Verification items for the finished model (mm, model axes). A direction names the side the tool comes from. Coordinates: 2 decimals unless noted, no trailing zeros. Write each loop counter-clockwise with the first axis right and the second up, starting at its lowest first coordinate (ties: lowest second). Pieces come first, ordered by that corner, then holes. Notation, with made-up numbers: (79, 7) -> (94, 7) arc R7 ccw to (94, 14) -> close; hole circle Ø4 at (8, -2). An arc over 180 degrees is marked (long way). Answer in a Markdown table with one row per item.
```python
from build123d import *

# Parameters (mm, degrees)
SKETCH1_R           = 1.3462
SKETCH1_W           = 3.7846
SKETCH1_H           = 52.6961
BOSS_EXTRUDE1_DEPTH = 3.048
SKETCH2_R           = 1.524
CUT_EXTRUDE1_DEPTH  = 430.898988368


with BuildPart() as part:
    # Sketch1 → Boss-Extrude1 (new body)
    # profile 1 of 3: a face of its own
    with BuildSketch(Plane.XY):
        with BuildLine():
            Line((-401.0571, 150.956597849), (-401.0571, 148.341))
            Line((-401.0571, 148.341), (-399.1521, 148.341))
            Line((-399.1521, 148.341), (-395.3675, 148.341))
            Line((-395.3675, 148.341), (-395.3675, 149.2432))
            Line((-395.3675, 149.2432), (-309.8086, 149.2432))
            Line((-309.8086, 149.2432), (-309.8086, 128.8851))
            Line((-309.8086, 128.8851), (-305.87795, 128.8851))
            Line((-305.87795, 128.8851), (-301.9473, 132.81575))
            Line((-301.9473, 132.81575), (-301.9473, 150.9704))
            ThreePointArc((-301.9473, 150.9704), (-303.063223164, 153.664476836), (-305.7573, 154.7804))
            Line((-305.7573, 154.7804), (-397.247125, 154.7804))
            ThreePointArc((-397.247125, 154.7804), (-399.946077222, 153.659592612), (-401.0571, 150.956597849))
        make_face()
        with Locations(Location((-397.247125, 150.9704, 0), (0, 0, 180))):
            Circle(SKETCH1_R, mode=Mode.SUBTRACT)
        with Locations(Location((-305.7573, 150.9704, 0), (0, 0, 180))):
            Circle(SKETCH1_R, mode=Mode.SUBTRACT)
    # profile 2 of 3: a face of its own
    with BuildSketch(Plane.XY):
        with Locations((-397.2598, 121.99295)):
            Rectangle(SKETCH1_W, SKETCH1_H)
    # profile 3 of 3: a face of its own
    with BuildSketch(Plane.XY):
        with BuildLine():
            Line((-395.3675, 95.6449), (-399.1521, 95.6449))
            Line((-399.1521, 95.6449), (-401.0571, 95.6449))
            Line((-401.0571, 95.6449), (-401.0571, 91.659304166))
            ThreePointArc((-401.0571, 91.659304166), (-399.951018769, 88.947400452), (-397.2472, 87.8217))
            Line((-397.2472, 87.8217), (-378.5565, 87.8217))
            Line((-378.5565, 87.8217), (-368.3165, 91.1883))
            Line((-368.3165, 91.1883), (-315.9973, 91.1883))
            Line((-315.9973, 91.1883), (-305.7573, 87.8217))
            ThreePointArc((-305.7573, 87.8217), (-303.063223164, 88.937623164), (-301.9473, 91.6317))
            Line((-301.9473, 91.6317), (-301.9473, 111.74645))
            Line((-301.9473, 111.74645), (-305.87795, 115.6771))
            Line((-305.87795, 115.6771), (-309.8086, 115.6771))
            Line((-309.8086, 115.6771), (-309.8086, 92.9525))
            Line((-309.8086, 92.9525), (-395.3675, 92.9525))
            Line((-395.3675, 92.9525), (-395.3675, 95.6449))
        make_face()
        with Locations(Location((-397.2472, 91.6317, 0), (0, 0, 180))):
            Circle(SKETCH1_R, mode=Mode.SUBTRACT)
        with Locations(Location((-305.7573, 91.6317, 0), (0, 0, 180))):
            Circle(SKETCH1_R, mode=Mode.SUBTRACT)
    extrude(amount=BOSS_EXTRUDE1_DEPTH)

    # Sketch2 → Cut-Extrude1 (cut, through all)
    with BuildSketch(Plane(origin=(0, 0, 0), x_dir=(-1, 0, 0), z_dir=(0, 0, -1))):
        with Locations((305.7573, 150.9704)):
            Circle(SKETCH2_R)
        with Locations((305.7573, 91.6317)):
            Circle(SKETCH2_R)
        with Locations((397.2472, 91.6317)):
            Circle(SKETCH2_R)
        with Locations((397.247125, 150.9704)):
            Circle(SKETCH2_R)
    extrude(amount=-CUT_EXTRUDE1_DEPTH, mode=Mode.SUBTRACT)


solid = part.part
```
1. Sectioned sample at C-C, the plane z = 0.55. Count the separate pieces of the cut face and the enclosed holes in it, and give its area (3 significant figures).
Findings below:
| item | result |
|---|---|
| separate pieces | 1 |
| enclosed holes | 4 |
| area | 1,350 mm² |
2. Material ranges on probe 1 along X at (y, z) = (102.5, 2.6); probe 2 along Y at (x, z) = (-339, 1.75); probe 3 along X at (y, z) = (129, 2.5), recorded low to high. Write a range as from..to.
Findings below:
| item | result |
|---|---|
| probe 1 | x = -399.15..-395.37, -309.81..-301.95 |
| probe 2 | y = 91.19..92.95, 149.24..154.78 |
| probe 3 | x = -399.15..-395.37, -309.81..-305.76 |
3. Access from +Z, -Z, +X, -X, +Y, -Y to the whole of each face (thin tool, end or side, straight path). Record for faces 4 (the face through (-353, 149.243, 2)), 5 (the face through (-400, 95.645, 2)), 6 (the face through (-308, 128.885, 2)), 7 (the face through (-388, 87.822, 2)), 8 (the face through (-373.51, 89.48, 1.5)).
Findings below:
| item | result |
|---|---|
| face 4 | +Z, -Z |
| face 5 | +Z, -Z, -X |
| face 6 | +Z, -Z, +X |
| face 7 | +Z, -Z, +X, -X, -Y |
| face 8 | +Z, -Z, -Y |
4. Sectioned sample at A-A, the plane x = -357.5. Record the cut outline in (y, z).
Findings below:
| item | result |
|---|---|
| outline | (91.19, 0) -> (92.95, 0) -> (92.95, 3.05) -> (91.19, 3.05) -> close; (149.24, 0) -> (154.78, 0) -> (154.78, 3.05) -> (149.24, 3.05) -> close |
5. Sectioned sample at D-D, the plane y = 122. Record the cut outline in (x, z).
Findings below:
| item | result |
|---|---|
| outline | (-399.15, 0) -> (-395.37, 0) -> (-395.37, 3.05) -> (-399.15, 3.05) -> close |
6. Go/stop test with flat-tipped pins: pin 1 (1.5 mm diameter, centred on x = -355, z = 2, fed in from -Y); pin 2 (0.6 mm diameter, centred on x = -399.5, z = 1, fed in from +Y); pin 3 (1 mm diameter, centred on y = 110, z = 2, fed in from -X). Record where each tip stops, or that it passes through.
Findings below:
| item | result |
|---|---|
| pin 1 | stops at y = 91.19 |
| pin 2 | stops at y = 154.24 |
| pin 3 | stops at x = -399.15 |
7. Sectioned sample at B-B, the plane y = 106.5. Record the cut outline in (x, z), and give its area (3 significant figures).
Findings below:
| item | result |
|---|---|
| outline | (-399.15, 0) -> (-395.37, 0) -> (-395.37, 3.05) -> (-399.15, 3.05) -> close; (-309.81, 0) -> (-301.95, 0) -> (-301.95, 3.05) -> (-309.81, 3.05) -> close |
| area | 35.5 mm² |
8. Release check for a two-part mould opening along X. For faces 1 (the face through (-307.165, 91.048, 1.503)), 2 (the face through (-348, 151, 3.048)), 3 (the face through (-399.152, 122, 2)) record: released by +X, released by -X, zero draft, split by the parting line, or undercut.
Findings below:
| item | result |
|---|---|
| face 1 | undercut |
| face 2 | zero draft |
| face 3 | released by -X |
